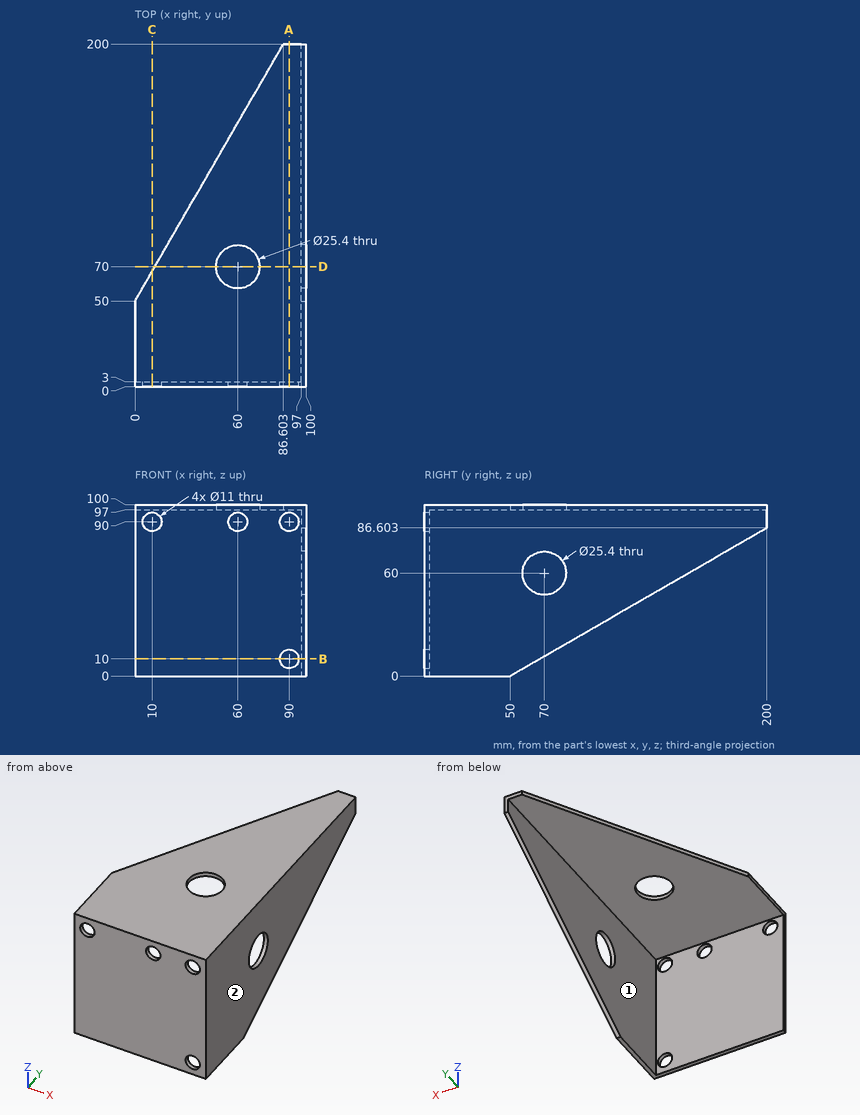
Could you check a few things on this drawing? It's one solid part, dimensions in mm from its lowest x, y, z. A direction names the side the tool comes from. Coordinates: 2 decimals unless noted, no trailing zeros. Order: outer loops, then holes, each group sorted by start corner. A loop starts at its lowest first (then second) coordinate and runs counter-clockwise, first axis right, second up. Notation, with made-up numbers: M 61,-23.5 L 82,-23.5 A20 ccw 82,-8.5 Z; hole C -0.5,40 d9. An arc over 180 degrees is marked long. Use a Markdown table: item, result. Add a question column.
Q1. I want a section at A-A on x = 90. List the corners of the cut face in (y, z) for me.
Q2. Which directions (+Z, -Z, +X, -X, +Y, -Y) give clear straight access to the entire face, cutting with the end or side of a thin tool? Please do the marked faces 1 and 2.
Q3. I want a section at D-D on y = 70. List the corners of the cut face in (x, z) for me.
Q4. I'm going to push a flat-ended pin straight in: pin 1 (12.5 mm diameter, centred on x = 10, z = 90, fed in from +Y). Where does the tip first touch, or does it pass through?
Q5. I want a section at C-C on x = 10. List the corners of the cut face in (y, z) for me.
Q6. If I drill on L1, parallel to Z at x = 60, y = 1.7; L2, parallel to Z at x = 74.5, y = 13; L3, parallel to Y at x = 30, z = 9, over which ranges is the centre line in solid material (lowest first)?
Q7. I want a section at B-B on z = 10. List the corners of the cut face in (x, y) for me.
Checked values:
| question | item | result |
|---|---|---|
| 1 | outline | M 0,0 L 3,0 L 3,4.5 L 0,4.5 Z; M 0,15.5 L 3,15.5 L 3,84.5 L 0,84.5 Z; M 0,95.5 L 3,95.5 L 3,97 L 200,97 L 200,100 L 0,100 Z |
| 2 | face 1 | -Z, -X, +Y |
| 2 | face 2 | +Z, -Z, +X, +Y, -Y |
| 3 | outline | M 11.55,97 L 47.3,97 L 47.3,100 L 11.55,100 Z; M 72.7,97 L 97,97 L 97,72.7 L 100,72.7 L 100,100 L 72.7,100 Z; M 97,11.55 L 100,11.55 L 100,47.3 L 97,47.3 Z |
| 4 | pin 1 | y = 3 |
| 5 | outline | M 0,0 L 3,0 L 3,84.5 L 0,84.5 Z; M 0,95.5 L 3,95.5 L 3,97 L 67.32,97 L 67.32,100 L 0,100 Z |
| 6 | L1 | 0 to 84.5, 95.5 to 100 |
| 6 | L2 | 97 to 100 |
| 6 | L3 | 0 to 3 |
| 7 | outline | M 0,0 L 84.5,0 L 84.5,3 L 0,3 Z; M 95.5,0 L 100,0 L 100,67.32 L 97,67.32 L 97,3 L 95.5,3 Z |
